Design review of the part shown in the three views and the two pictorial views. Dimensions are in mm from the part's minimum x, y and z. Round coordinates to 2 decimals unless told otherwise and drop trailing zeros. Loops run counter-clockwise (first coordinate to the right, second up) from the corner with the lowest first, then second, coordinate; pieces in that order, holes last. Notation, with made-up numbers: (-3, 15.25) -> (17, 15.25) arc R26 cw to (17, 42.25) -> close; hole circle Ø11 at (80.5, 57.5). An arc over 180 degrees is marked (long way). Return JSON: item names as keys, results as strings. Group by question number.
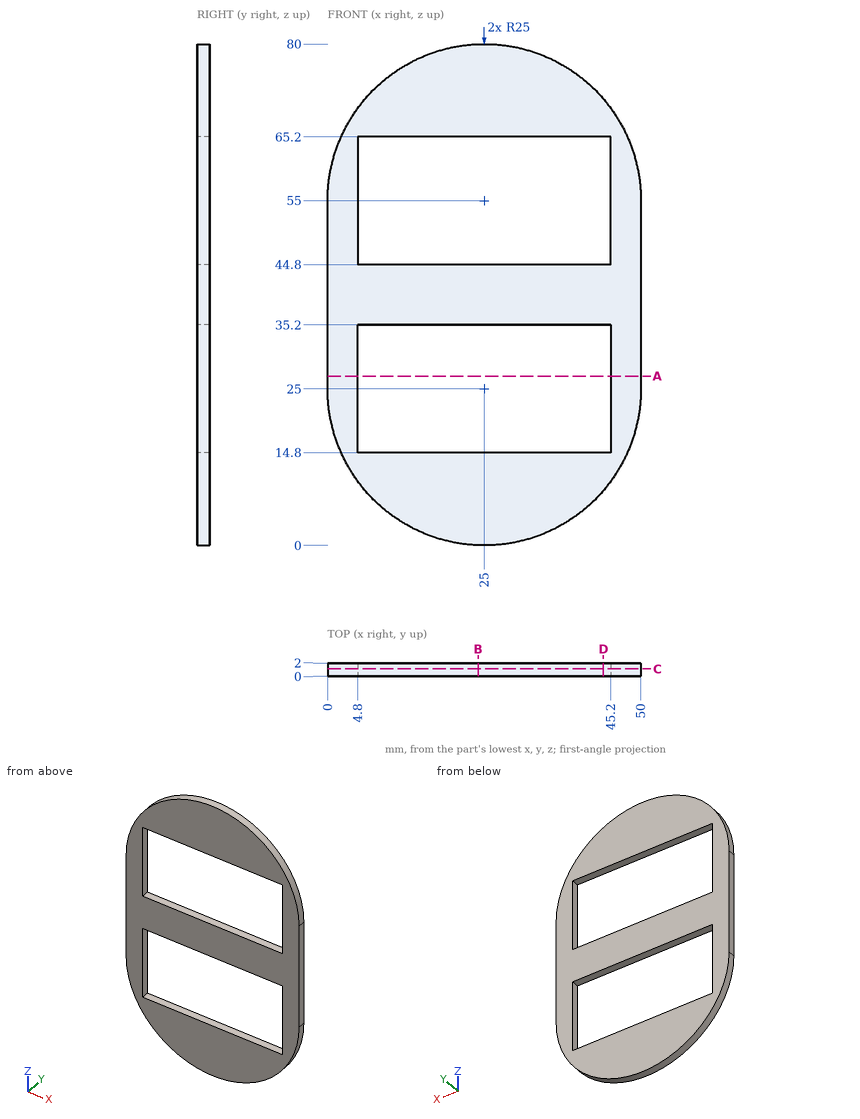
1. For P1, Ø1.5, axis at x = 19, z = 33, coming from the -Y side; P2, Ø1, axis at x = 18.5, y = 1.5, coming from the +Z side; P3, Ø0.6, axis at x = 26.5, y = 1, coming from the -Z side; P4, Ø1, axis at x = 16.5, y = 1.5, coming from the -Z side, all flat-tipped, find the tip position at first contact; note any pin that passes through.
2. We need section B-B, the plane x = 24. Write out the cut boundary in (y, z).
3. We need section D-D, the plane x = 44. Write out the cut boundary in (y, z), then the cut area to 3 significant figures.
4. We need section A-A, the plane z = 27. Write out the cut boundary in (x, y).
5. Wall thickness on line 1 (Z direction, x = 25, y = 1.25); line 2 (X direction, y = 1.7, z = 24.5) (3 decimals); line 3 (Z direction, x = 43, y = 1.6): over which ranges is each line inside the solid? List them lowest first.
6. We need section C-C, the plane y = 1.15. Write out the cut boundary in (x, z).
Check sheet entries:
{
 "1": {"P1": "passes through", "P2": "stops at z = 79.27", "P3": "stops at z = 0.03", "P4": "stops at z = 1.31"},
 "2": {"outline": "(0, 0.02) -> (2, 0.02) -> (2, 14.8) -> (0, 14.8) -> close; (0, 35.2) -> (2, 35.2) -> (2, 44.8) -> (0, 44.8) -> close; (0, 65.2) -> (2, 65.2) -> (2, 79.98) -> (0, 79.98) -> close"},
 "3": {"outline": "(0, 8.75) -> (2, 8.75) -> (2, 14.8) -> (0, 14.8) -> close; (0, 35.2) -> (2, 35.2) -> (2, 44.8) -> (0, 44.8) -> close; (0, 65.2) -> (2, 65.2) -> (2, 71.25) -> (0, 71.25) -> close", "area": "43.4 mm²"},
 "4": {"outline": "(0, 0) -> (4.8, 0) -> (4.8, 2) -> (0, 2) -> close; (45.2, 0) -> (50, 0) -> (50, 2) -> (45.2, 2) -> close"},
 "5": {"line 1": "z = 0 to 14.8, 35.2 to 44.8, 65.2 to 80", "line 2": "x = 0.005 to 4.8, 45.2 to 49.995", "line 3": "z = 7.65 to 14.8, 35.2 to 44.8, 65.2 to 72.35"},
 "6": {"outline": "(0, 25) arc R25 ccw to (50, 25) -> (50, 55) arc R25 ccw to (0, 55) -> close; hole (4.8, 14.8) -> (45.2, 14.8) -> (45.2, 35.2) -> (4.8, 35.2) -> close; hole (4.8, 44.8) -> (45.2, 44.8) -> (45.2, 65.2) -> (4.8, 65.2) -> close"}
}
